Can you work these out from the model? Positions are in its coordinate system, mm. Face numbers are marked on the shaded views. A direction names the side the tool comes from. Give positions to 0.01 mm unless a question says otherwise; leave off trailing zeros. Order: outer loops, then holes, each group sorted by start corner. A loop starts at its lowest first (then second) coordinate and runs counter-clockwise, first axis right, second up.
Item 1: If I drill on line 1 along X through (y, z) = (5.25, 15.5); line 2 along X through (y, z) = (10.25, 8); line 3 along X through (y, z) = (8, 3.75), over which ranges is the centre line in solid material (lowest first)?
Item 2: If we mould it in two halves opening along X, with no side actions, what happens to the marked faces 1, 2 and 3? For each: +X half, -X half, draft (parallel to the pull), parting line (faces both ways), or undercut.
Item 3: I'm going to push flat-ended pins straight in: pin 1 Ø4 at (y, z) = (4.5, 3) entering from +X; pin 2 Ø4 at (x, z) = (37, 5) entering from -Y; pin 3 Ø9 at (x, y) = (14.5, 6) entering from +Z. Where does each tip first touch, or does it pass through?
Item 4: I want a section at A-A, the plane y = 2.75. Write out the boundary of the cut face in (x, z).
Item 5: Which directions (+Z, -Z, +X, -X, +Y, -Y) give clear straight access to the entire face, cutting with the end or side of a thin tool? Please do the marked faces 4 and 5.
Item 6: I want a section at C-C, the plane y = 17.5. Write out the boundary of the cut face in (x, z).
Item 7: I want a section at B-B, the plane x = 37.5. Write out the boundary of the cut face in (y, z), then the cut area to 4 significant figures.
```python
from build123d import *

# Parameters (mm, degrees)
F1_DEPTH = 22.5
F2_W     = 10
F2_H     = 10
F3_DEPTH = 7.5
F4_SIZE  = 5
F6_R     = 3
F7_DEPTH = 29.584648


with BuildPart() as f1:
    # F0 (on Front) → F1 (new body)
    with BuildSketch(Plane.XZ):
        Polygon((0, 20), (0, 0), (43, 0), (43, 7.5), (25.5, 7.5), (25.5, 15), (7.5, 15), (7.5, 20), align=None)
    extrude(amount=-F1_DEPTH)

    # F2 (on face) → F3 (cut, through all)
    with BuildSketch(Plane.XY.offset(7.5)):
        with Locations((38, 5)):
            Rectangle(F2_W, F2_H)
    extrude(amount=-F3_DEPTH, mode=Mode.SUBTRACT)

    # F4
    f4_edges = [f1.edges().sort_by_distance(p)[0] for p in [
        (0, 11.25, 0),
    ]]
    chamfer(f4_edges, length=F4_SIZE)

    # F6 (on face) → F7 (cut, through all)
    with BuildSketch(Plane(origin=(25.620191, 0, 14.791824), x_dir=(0, 1, 0), z_dir=(0.866025, 0, 0.5))):
        with Locations((10.281982, 0)):
            Circle(F6_R)
    extrude(amount=-F7_DEPTH, mode=Mode.SUBTRACT)


solid = f1.part
```
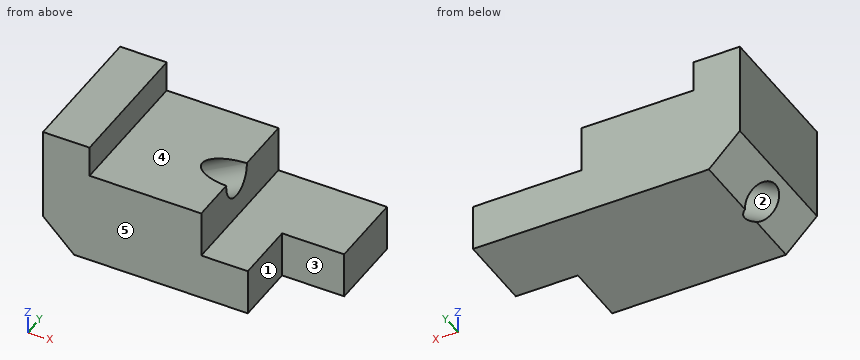
Results list:
1. line 1: x = 0 to 7.5
1. line 2: x = 0 to 7.86, 19.86 to 25.5
1. line 3: x = 1.25 to 2.6, 10.39 to 33
2. face 1: +X half
2. face 2: undercut
2. face 3: draft
3. pin 1: stops at x = 33
3. pin 2: stops at y = 10
3. pin 3: stops at z = 15
4. outline: (0, 5) - (5, 0) - (33, 0) - (33, 7.5) - (25.5, 7.5) - (25.5, 15) - (7.5, 15) - (7.5, 20) - (0, 20) - close
5. face 4: +Z, +X, +Y, -Y
5. face 5: +Z, -Z, +X, -X, -Y
6. outline: (0, 5) - (5, 0) - (43, 0) - (43, 7.5) - (25.5, 7.5) - (25.5, 15) - (7.5, 15) - (7.5, 20) - (0, 20) - close
7. outline: (10, 0) - (22.5, 0) - (22.5, 7.5) - (10, 7.5) - close
7. area: 93.75 mm2
